Geometry: final body of the model. Coordinates: model frame, mm. A direction names the side the tool comes from. Give positions to 0.01 mm unless a question says otherwise; leave off trailing zeros. Write each loop counter-clockwise with the first axis right and the second up, starting at its lowest first coordinate (ties: lowest second). Pieces come first, ordered by that corner, then holes. Notation, with made-up numbers: M 76,-14.5 L 80,-14.5 A8 cw 80,-1.5 Z; hole C 55.25,-23 d3. An arc over 180 degrees is marked long. Use one line per item in the form item = value. Start each with the question number.
Item 1: Pull-direction query (X, two-part tool) for faces 1 (the flat face through (-0.06, -460.03, 11.35)), 2 (the flat face through (0, -6, -11.112)), 3 (the flat face through (12.7, -6, 0)); classes: released by +X, released by -X, zero draft, split by the parting line, or undercut.
Item 2: Access query for faces 4 (the flat face through (0, -6, 12.7)), 5 (the flat face through (11.112, -6, 0)). Directions: +Z, -Z, +X, -X, +Y, -Y. A direction counts if a zero-diameter tool reaches every point of the face in a straight line with its end or side. Return the directions, or none.
Item 3: Section query A-A on z = 6.25. Return loops of the section in (x, y), then the cut area to 3 significant figures.
Item 4: Section query B-B on x = 2.25. Return loops of the section in (y, z).
Item 5: Section query C-C on y = 3. Return loops of the section in (x, z), then the cut area to 3 significant figures.
Item 6: Material intervals for line 1 along X through (y, z) = (-418.5, 7.25); line 2 along Y through (x, z) = (-11.5, 3), sorted ascending. Write a range as from..to.
from build123d import *

# Parameters (mm, degrees)
F0_W     = 25.4
F0_H     = 25.4
F0_W_2   = 22.225
F0_H_2   = 22.225
F1_DEPTH = 462.28
F3_DEPTH = 25.401


# Not quite as in the source:
# - a pattern or mirror of a feature is missing from the dataset's text; its kind, count and spacing are read off the source's solid


with BuildPart() as f1:
    # F0 (on Front) → F1 (new body, symmetric)
    with BuildSketch(Plane.XZ):
        Rectangle(F0_W, F0_H)
        Rectangle(F0_W_2, F0_H_2, mode=Mode.SUBTRACT)
    extrude(amount=F1_DEPTH, both=True)

    # F2 (on face) → F3 (cut, through all)
    with BuildSketch(Plane.XY.offset(12.7)):
        Polygon((12.7, 462.28), (-12.7, 462.28), (-12.7, 457.80129469), align=None)
    f3 = extrude(amount=-F3_DEPTH, mode=Mode.SUBTRACT)

    # F3_copies: F3 across plane
    add(f3.mirror(Plane(origin=(0, 0, 0), x_dir=(0, 0, -1), z_dir=(0, -1, 0))), mode=Mode.SUBTRACT)


solid = f1.part
Answer sheet:
q1.face_1 = released by -X
q1.face_2 = undercut
q1.face_3 = released by +X
q2.face_4 = +Z, +X, -X, +Y, -Y
q2.face_5 = +Y, -Y
q3.outline = M -12.7,-457.8 L -11.11,-458.08 L -11.11,458.08 L -12.7,457.8 Z; M 11.11,-462 L 12.7,-462.28 L 12.7,462.28 L 11.11,462 Z
q3.area = 2,920 mm2
q4.outline = M -460.44,-12.7 L 460.44,-12.7 L 460.44,-11.11 L -460.44,-11.11 Z; M -460.44,11.11 L 460.44,11.11 L 460.44,12.7 L -460.44,12.7 Z
q5.outline = M -12.7,-12.7 L 12.7,-12.7 L 12.7,12.7 L -12.7,12.7 Z; hole M -11.11,-11.11 L 11.11,-11.11 L 11.11,11.11 L -11.11,11.11 Z
q5.area = 151 mm2
q6.line_1 = -12.7..-11.11, 11.11..12.7
q6.line_2 = -458.01..458.01
